Geometry: see drawing. Coordinates: mm, zero at the bounding-box minimum. A direction names the side the tool comes from. Round coordinates to 2 decimals unless told otherwise and drop trailing zeros. Loops run counter-clockwise (first coordinate to the right, second up) from the corner with the lowest first, then second, coordinate; pieces in that order, holes last. Notation, with made-up numbers: (76.25, 75.25) - (83.25, 75.25) arc R21 cw to (83.25, 89.25) - close; hole circle Ø9 at (50.5, 30). An arc over 180 degrees is marked (long way). Use CSV: the item, a comma, the result in double quotes. Start each with the question number.
1. Access query for the marked faces 1, 2 and 3. Directions: +Z, -Z, +X, -X, +Y, -Y. A direction counts if a zero-diameter tool reaches every point of the face in a straight line with its end or side. Return the directions, or none.
2. Cut plane A-A (y = 17.5). Return loops of the section in (x, z).
3. Material intervals for probe 1 along Y at (x, z) = (43, 33.05); probe 2 along Y at (x, z) = (18, 32.85); probe 3 along Z at (x, y) = (37, 10), sorted ascending. Write a range as from..to.
4. Pin query (flat end, axial travel): P1, Ø0.9, axis at y = 37, z = 14.5, coming from the +X side; P2, Ø4, axis at x = 20, z = 14.5, coming from the -Y side; P3, Ø8, axis at x = 43, y = 7.5, coming from the +Z side; P4, Ø11.5, axis at x = 22.5, y = 10, coming from the -Z side. Return the tip coordinate at first contact, or that it passes through.
5. Cut plane D-D (x = 43). Return loops of the section in (y, z), and give its area (3 significant figures).
6. Cut plane C-C (z = 5). Return loops of the section in (x, y).
7. Pull-direction query (X, two-part tool) for the marked faces 4, 5 and 6; classes: +X half, -X half, draft (parallel to the pull), parting line (faces both ways), or undercut.
8. Cut plane B-B (x = 18). Return loops of the section in (y, z).
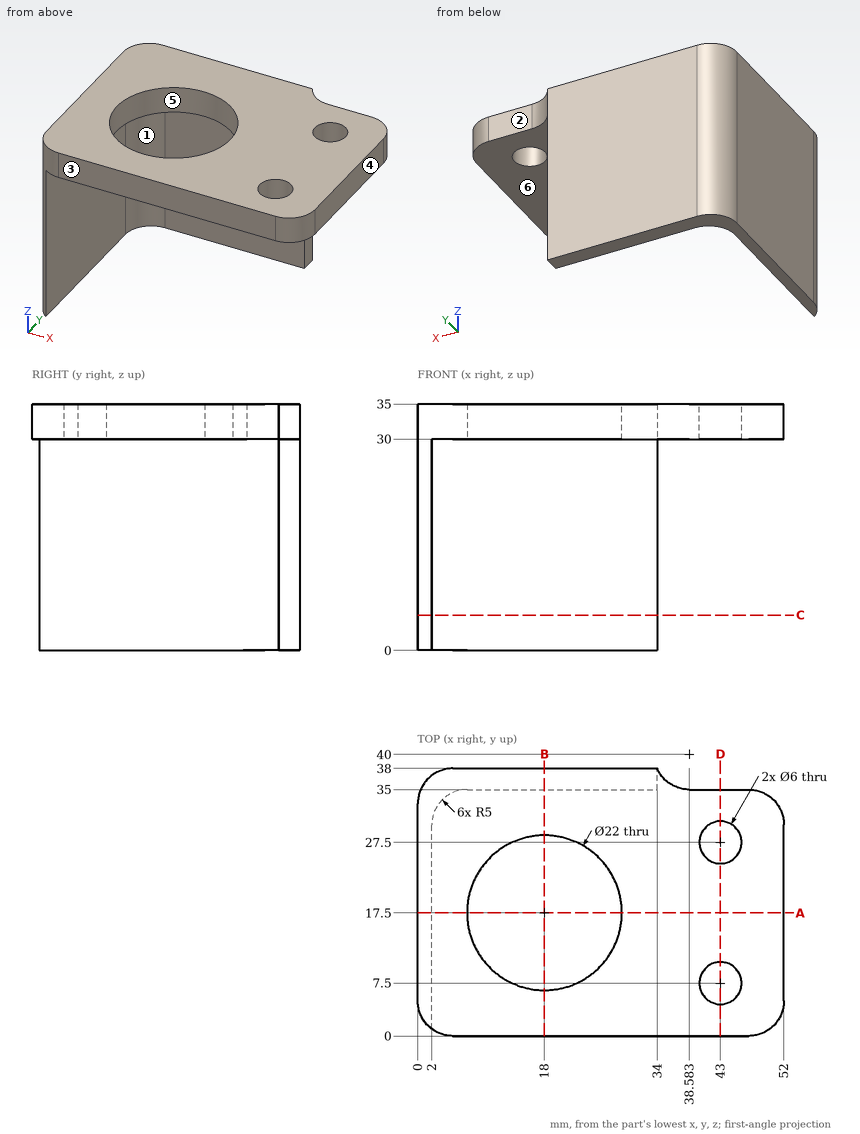
Established:
1,face 1,"-Z, +X, -Y"
1,face 2,"+Z, -Z, +X, +Y"
1,face 3,"+Z, -Z, +X, -X, -Y"
2,outline,"(0, 0) - (2, 0) - (2, 30) - (7, 30) - (7, 35) - (0, 35) - close; (29, 30) - (52, 30) - (52, 35) - (29, 35) - close"
3,probe 1,"y = 0..4.5, 10.5..24.5, 30.5..35"
3,probe 2,"y = 0..6.5, 28.5..38"
3,probe 3,"z = 30..35"
4,P1,"stops at x = 34"
4,P2,"stops at y = 35"
4,P3,"stops at z = 35"
4,P4,"stops at z = 30"
5,outline,"(0, 30) - (4.5, 30) - (4.5, 35) - (0, 35) - close; (10.5, 30) - (24.5, 30) - (24.5, 35) - (10.5, 35) - close; (30.5, 30) - (35, 30) - (35, 35) - (30.5, 35) - close"
5,area,"115 mm2"
6,outline,"(0, 5) arc R5 ccw to (2, 1) - (2, 30) arc R5 cw to (7, 35) - (34, 35) - (34, 38) - (5, 38) arc R5 ccw to (0, 33) - close"
7,face 4,"+X half"
7,face 5,"undercut"
7,face 6,"draft"
8,outline,"(0, 30) - (6.5, 30) - (6.5, 35) - (0, 35) - close; (28.5, 30) - (35, 30) - (35, 0) - (38, 0) - (38, 35) - (28.5, 35) - close"
